Build history of the part. All positions in model axes, mm. A direction names the side the tool comes from. Round coordinates to 2 decimals unless told otherwise and drop trailing zeros. Write each loop counter-clockwise with the first axis right and the second up, starting at its lowest first coordinate (ties: lowest second). Pieces come first, ordered by that corner, then holes. Notation, with made-up numbers: M 48,27.25 L 52,27.25 A23 cw 52,61.25 Z; hole C 22.25,5.25 d10. An arc over 180 degrees is marked long. One line per item, written item: value. Start each with the question number.
Autodesk Inventor part; units mm, degrees
ref_plane "YZ Plane" through (0, 0, 0) normal (1, 0, 0) x (0, 1, 0)
ref_plane "XZ Plane" through (0, 0, 0) normal (0, 1, 0) x (-1, 0, 0)
ref_plane "XY Plane" through (0, 0, 0) normal (0, 0, 1) x (1, 0, 0)
sketch "Boceto1" plane through (0, 0, 0) normal (0, 1, 0) x (-1, 0, 0)
  circle A0 centre (0, 0) radius 9
  dimension "d0" = 18
extrude "Extrusión1" add sketch "Boceto1" along normal blind 38
sketch "Boceto2" plane through (0, 38, 0) normal (0, 1, 0) x (1, 0, 0)
  circle A0 centre (0, 0) radius 12
  dimension "d3" = 24
extrude "Extrusión2" add sketch "Boceto2" along normal blind 154
sketch "Boceto3" plane through (0, 0, 0) normal (0, 0, 1) x (1, 0, 0)
  line L0 (0, 0) -> (0, 203) construction
  circle A0 centre (0, 203) radius 4
  arc A1 (10, 203) -> (-10, 203) centre (0, 203) ccw
  line L1 (10, 203) -> (10, 192)
  line L2 (12, 192) -> (-12, 192)
  line L3 (-10, 192) -> (-10, 203)
  line L4 (-10, 192) -> (10, 192)
  dimension "d6" = 203
  dimension "d7" = 8
  dimension "d8" = 20
  dimension "d9" = 20
extrude "Extrusión3" add sketch "Boceto3" along normal mid plane 13
sketch "Boceto4" plane through (0, 0, 0) normal (0, 0, 1) x (1, 0, 0)
  line L0 (0, 0) -> (0, 3.8) construction
  line L1 (0, 3.8) -> (9, 3.8) construction
  line L2 (9, 0) -> (9, 38)
  line L3 (9, 3.8) -> (9, 2.3)
  line L4 (9, 2.3) -> (8.5, 2.3)
  line L5 (8.5, 2.3) -> (8.5, 3.8)
  line L6 (8.5, 3.8) -> (9, 3.8)
  dimension "d12" = 3.8
  dimension "d13" = 1.5
  dimension "d14" = 0.5
revolve "Revolución1" cut sketch "Boceto4" angle 360 about axis through (0, 0, 0) along (0, 1, 0)
chamfer "Chaflán1" distance 1 angle 45 1 edges at (9, 0, 0) measured on face at (-2.2455, 0, -1.9894)
properties part number "14_Eje"
Item 1: Drop flat-ended pins along their axis: pin 1 (5 mm diameter, centred on x = 0, y = 203, fed in from +Z); pin 2 (2 mm diameter, centred on y = 46, z = -7, fed in from +X); pin 3 (2 mm diameter, centred on y = 48, z = -2.5, fed in from -X); pin 4 (12 mm diameter, centred on x = 8.5, y = 55, fed in from -Z). Give the stop position or say it passes through.
Item 2: Cut at D-D, the plane y = 194. Write the cut outline in (x, z).
Item 3: Cut at C-C, the plane y = 54. Write the cut outline in (x, z), plus the area to 3 significant figures.
Item 4: Which spindle directions (+Z, -Z, +X, -X, +Y, -Y) get a long thin tool onto all of the face, cutting with end or side? Do faces 1 (the flat face through (0, 198, -6.5)), 2 (the cylindrical face through (1.172, 20.661, -8.923)), 3 (the flat face through (10, 198, 0)), 4 (the flat face through (8, 2.3, 3.3)). Say none if no direction does.
Item 5: Cut at A-A, the plane x = 0. Write the cut outline in (y, z), plus the area to 3 significant figures.
Item 6: Cut at B-B, the plane z = 0. Write the cut outline in (x, y), plus the area to 3 significant figures.
Item 7: Drill centre lines: line 1 (Y direction, x = 0, z = 3.75); line 2 (Z direction, x = 0, y = 176); line 3 (Y direction, x = 10.25, z = -2.75). Where is each one in solid material? Low to high.
Item 8: Two-plate mould, pull along Y, no slides. Class faces 5 (the flat face through (0, 198, 6.5)), 6 (the cylindrical face through (4.57, 3.06, -7.167)), 7 (the cylindrical face through (-0.521, 199.034, -0.091)), 8 (the flat face through (0, 0, 0)): pulls with the +Y half, pulls with the -Y half, needs draft (parallel to the pull), parting line crosses it, or undercut.
Computed values:
1. pin 1: passes through
1. pin 2: stops at x = 10.39
1. pin 3: stops at x = -11.91
1. pin 4: stops at z = -11.74
2. outline: M -10,-6.5 L 10,-6.5 L 10,6.5 L -10,6.5 Z
3. outline: C 0,0 d24
3. area: 452 mm2
4. face 1: -Z, +X, -X, +Y
4. face 2: -Y
4. face 3: +Z, -Z, +X, +Y
4. face 4: none
5. outline: M 0,-8 L 1,-9 L 2.3,-9 L 2.3,-8.5 L 3.8,-8.5 L 3.8,-9 L 38,-9 L 38,-12 L 192,-12 L 192,-6.5 L 199,-6.5 L 199,6.5 L 192,6.5 L 192,12 L 38,12 L 38,9 L 3.8,9 L 3.8,8.5 L 2.3,8.5 L 2.3,9 L 1,9 L 0,8 Z; M 207,-6.5 L 213,-6.5 L 213,6.5 L 207,6.5 Z
5. area: 4,550 mm2
6. outline: M -12,38 L -9,38 L -9,3.8 L -8.5,3.8 L -8.5,2.3 L -9,2.3 L -9,1 L -8,0 L 8,0 L 9,1 L 9,2.3 L 8.5,2.3 L 8.5,3.8 L 9,3.8 L 9,38 L 12,38 L 12,192 L 10,192 L 10,203 A10 ccw -10,203 L -10,192 L -12,192 Z; hole C 0,203 d8
6. area: 4,700 mm2
7. line 1: y = 0 to 199, 207 to 213
7. line 2: z = -12 to 12
7. line 3: y = 38 to 192
8. face 5: needs draft
8. face 6: undercut
8. face 7: undercut
8. face 8: pulls with the -Y half
